Source: three-view drawing plus pictorial views. Frame: mm from the lowest corner of the part. Give positions to 0.01 mm unless a question says otherwise; leave off trailing zeros. Order: outer loops, then holes, each group sorted by start corner. A loop starts at its lowest first (then second) coordinate and runs counter-clockwise, first axis right, second up. Notation, with made-up numbers: (87, 86.25) -> (117, 86.25) arc R25 ccw to (117, 103.25) -> close; hole circle Ø9 at (-33.5, 18.25). An arc over 180 degrees is marked (long way). Use a Markdown table: item, result. Add a question column.
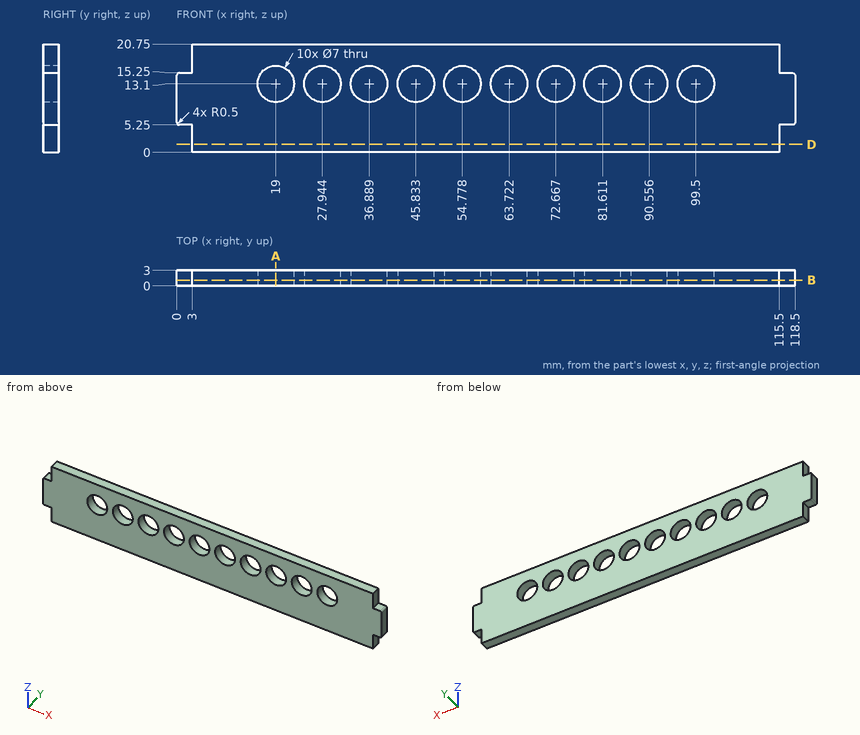
Q1. Section query B-B (y = 1.1). Give the number of separate pieces and of enclosed holes in the cut face, plus the area to 3 significant figures.
Q2. First-contact query: pin 1 (1.5 mm diameter, centred on y = 1, z = 17, fed in from +X); pin 2 (1.2 mm diameter, centred on x = 116.5, y = 1.5, fed in from +Z). Flat tips, straight axial feed; report the tip coordinate or a pass-through.
Q3. Section query A-A (x = 19). Return loops of the section in (y, z).
Q4. Ray query, line 1 (Z direction, x = 72.5, y = 2.5); line 2 (X direction, y = 0.7, z = 4); line 3 (X direction, y = 0.5, z = 5.5) (1 decimal). Return the intervals inside material, ascending.
Q5. Section query D-D (z = 1.5). Return loops of the section in (x, y).
Solution:
| question | item | result |
|---|---|---|
| 1 | separate pieces | 1 |
| 1 | enclosed holes | 10 |
| 1 | area | 2,010 mm² |
| 2 | pin 1 | stops at x = 115.5 |
| 2 | pin 2 | stops at z = 15.25 |
| 3 | outline | (0, 0) -> (3, 0) -> (3, 9.6) -> (0, 9.6) -> close; (0, 16.6) -> (3, 16.6) -> (3, 20.75) -> (0, 20.75) -> close |
| 4 | line 1 | z = 0 to 9.6, 16.6 to 20.75 |
| 4 | line 2 | x = 3 to 115.5 |
| 4 | line 3 | x = 0.1 to 118.4 |
| 5 | outline | (3, 0) -> (115.5, 0) -> (115.5, 3) -> (3, 3) -> close |
